from build123d import *

# Parameters (mm, degrees)
SKETCH1_W           = 127
SKETCH1_H           = 101.6
BOSS_EXTRUDE1_DEPTH = 7.62
SKETCH3_W           = 38.1
SKETCH3_H           = 101.6
BOSS_EXTRUDE2_DEPTH = 3.81
SKETCH4_W           = 25.4
SKETCH4_H           = 31.75
CUT_EXTRUDE1_DEPTH  = 7.62
FILLET1_R           = 17.78
BOSS_EXTRUDE3_DEPTH = 10.16
SKETCH6_W           = 1.401774382
SKETCH6_H           = 7.084034581
SKETCH6_W_2         = 1.657965541
SKETCH6_W_3         = 0.723515752
SKETCH6_W_4         = 1.5072414
SKETCH6_W_5         = 1.65796554
SKETCH6_W_6         = 12.660827761
SKETCH6_H_2         = 4.394326049
SKETCH6_W_7         = 12.660827762
BOSS_EXTRUDE4_DEPTH = 5.08
SKETCH7_W           = 0.989162869
SKETCH7_H           = 4.394326049
SKETCH7_W_2         = 1.219468424
CUT_EXTRUDE2_DEPTH  = 5.08
SKETCH8_W           = 20.126718604
SKETCH8_H           = 7.896323228
BOSS_EXTRUDE5_DEPTH = 2.54
SKETCH9_W           = 0.213588314
SKETCH9_H           = 99.880159493
BOSS_EXTRUDE6_DEPTH = 2.54


with BuildPart() as part:
    # Sketch1 → Boss-Extrude1 (new body)
    with BuildSketch(Plane.XY):
        with Locations((63.5, 50.8)):
            Rectangle(SKETCH1_W, SKETCH1_H)
    extrude(amount=BOSS_EXTRUDE1_DEPTH)

    # Sketch3 → Boss-Extrude2 (add)
    with BuildSketch(Plane(origin=(0, 0, 0), x_dir=(-1, 0, 0), z_dir=(0, 0, -1))):
        with Locations((-63.5, 50.8)):
            Rectangle(SKETCH3_W, SKETCH3_H)
    extrude(amount=BOSS_EXTRUDE2_DEPTH)

    # Sketch4 → Cut-Extrude1 (cut)
    with BuildSketch(Plane(origin=(0, 0, 0), x_dir=(-1, 0, 0), z_dir=(0, 0, -1))):
        with Locations((-25.4, 76.835)):
            Rectangle(SKETCH4_W, SKETCH4_H)
        with Locations((-107.95, 76.835)):
            Rectangle(SKETCH4_W, SKETCH4_H)
    extrude(amount=-CUT_EXTRUDE1_DEPTH, mode=Mode.SUBTRACT)

    # Fillet1
    fillet1_edges = [part.edges().sort_by_distance(p)[0] for p in [
        (127, 0, 3.81),
        (0, 0, 3.81),
    ]]
    fillet(fillet1_edges, radius=FILLET1_R)

    # Sketch5 → Boss-Extrude3 (add)
    with BuildSketch(Plane.XZ):
        Polygon((43.18, 7.62), (52.463035847, 23.698689735), (74.536964153, 23.698689735), (83.82, 7.62), align=None)
    extrude(amount=-BOSS_EXTRUDE3_DEPTH)

    # Sketch6 → Boss-Extrude4 (add)
    with BuildSketch(Plane.XZ):
        with Locations((54.433923038, 19.138517409)):
            Rectangle(SKETCH6_W, SKETCH6_H)
        with Locations((58.82755166, 19.138517409)):
            Rectangle(SKETCH6_W_2, SKETCH6_H)
        with Locations((63.515052474, 19.138517409)):
            Rectangle(SKETCH6_W_3, SKETCH6_H)
        with Locations((66.13767245, 19.138517409)):
            Rectangle(SKETCH6_W_4, SKETCH6_H)
        with Locations((69.528965601, 19.138517409)):
            Rectangle(SKETCH6_W_5, SKETCH6_H)
        with Locations((57.99856889, 9.353111302)):
            Rectangle(SKETCH6_W_6, SKETCH6_H_2)
        with Locations((70.659396651, 9.353111302)):
            Rectangle(SKETCH6_W_7, SKETCH6_H_2)
    extrude(amount=BOSS_EXTRUDE4_DEPTH)

    # Sketch7 → Cut-Extrude2 (cut)
    with BuildSketch(Plane.XZ.offset(5.08)):
        with Locations((63.834401336, 9.353111302)):
            Rectangle(SKETCH7_W, SKETCH7_H)
        with Locations((64.938716982, 9.353111302)):
            Rectangle(SKETCH7_W_2, SKETCH7_H)
    extrude(amount=-CUT_EXTRUDE2_DEPTH, mode=Mode.SUBTRACT)

    # Sketch8 → Boss-Extrude5 (add)
    with BuildSketch(Plane.XZ):
        with Locations((62.814636368, 19.241529297)):
            Rectangle(SKETCH8_W, SKETCH8_H)
    extrude(amount=BOSS_EXTRUDE5_DEPTH)

    # Sketch9 → Boss-Extrude6 (add)
    with BuildSketch(Plane.XY.offset(7.62)):
        with Locations((18.943205843, 49.940079747)):
            Rectangle(SKETCH9_W, SKETCH9_H)
    extrude(amount=BOSS_EXTRUDE6_DEPTH)


solid = part.part
Part model, mm, in its own coordinate system. A direction names the side the tool comes from. Coordinates: 2 decimals unless noted, no trailing zeros. Order: outer loops, then holes, each group sorted by start corner. A loop starts at its lowest first (then second) coordinate and runs counter-clockwise, first axis right, second up.
(1) Pull direction X, two halves, no side cores. Call faces 4 (the face through (127, 59, 4)), 5 (the face through (51.668, -3, 9)), 6 (the face through (68.7, -4, 19)): pulls with the +X half, pulls with the -X half, needs draft (parallel to the pull), parting line crosses it, or undercut.
Check sheet entries:
face 4: pulls with the +X half
face 5: pulls with the -X half
face 6: undercut
(2) Slice it at D-D, the plane y = 24. Write the cut outline in (x, z), and give its area (3 significant figures).
Check sheet entries:
outline: (0, 0) - (44.45, 0) - (44.45, -3.81) - (82.55, -3.81) - (82.55, 0) - (127, 0) - (127, 7.62) - (19.05, 7.62) - (19.05, 10.16) - (18.84, 10.16) - (18.84, 7.62) - (0, 7.62) - close
area: 1,110 mm2
(3) Slice it at B-B, the plane x = 23. Write the cut outline in (y, z), and give its area (3 significant figures).
Check sheet entries:
outline: (0, 0) - (60.96, 0) - (60.96, 7.62) - (0, 7.62) - close; (92.71, 0) - (101.6, 0) - (101.6, 7.62) - (92.71, 7.62) - close
area: 532 mm2
(4) Probe L1, parallel to X at y = 74, z = 6.5; L2, parallel to Y at x = 87, z = 4.5; L3, parallel to Y at x = 26.5, z = 1. List the from-to ranges inside material, lowest first.
Check sheet entries:
L1: x = 0 to 12.7, 38.1 to 95.25, 120.65 to 127
L2: y = 0 to 101.6
L3: y = 0 to 60.96, 92.71 to 101.6
(5) Slice it at C-C, the plane z = 5. Write the cut outline in (x, y), and give its area (3 significant figures).
Check sheet entries:
outline: (0, 17.78) arc R17.78 ccw to (17.78, 0) - (109.22, 0) arc R17.78 ccw to (127, 17.78) - (127, 101.6) - (0, 101.6) - close; hole (12.7, 60.96) - (38.1, 60.96) - (38.1, 92.71) - (12.7, 92.71) - close; hole (95.25, 60.96) - (120.65, 60.96) - (120.65, 92.71) - (95.25, 92.71) - close
area: 11,200 mm2
(6) Tool access for faces 1 (the face through (104, 52, 0)), 2 (the face through (59.657, -4, 19)), 3 (the face through (108, 92.71, 4)): list every direction of +Z, -Z, +X, -X, +Y, -Y with a clear straight run to the whole face (end or side of a thin tool).
Check sheet entries:
face 1: -Z, +X, +Y, -Y
face 2: +Z, -Y
face 3: +Z, -Z
(7) Slice it at A-A, the plane y = 87. Write the cut outline in (x, z), and give its area (3 significant figures).
Check sheet entries:
outline: (0, 0) - (12.7, 0) - (12.7, 7.62) - (0, 7.62) - close; (18.84, 7.62) - (19.05, 7.62) - (19.05, 10.16) - (18.84, 10.16) - close; (38.1, 0) - (44.45, 0) - (44.45, -3.81) - (82.55, -3.81) - (82.55, 0) - (95.25, 0) - (95.25, 7.62) - (38.1, 7.62) - close; (120.65, 0) - (127, 0) - (127, 7.62) - (120.65, 7.62) - close
area: 726 mm2
(8) Pin check, flat tips, straight feed: pin 1 Ø12 at (y, z) = (26, 16) entering from -X; pin 2 Ø5.5 at (x, y) = (71, -2.5) entering from +Z; pin 3 Ø2 at (y, z) = (-4, 18) entering from -X; pin 4 Ø12 at (y, z) = (10, 9.5) entering from -X. Stop position of each tip, or through.
Check sheet entries:
pin 1: stops at x = 18.84
pin 2: stops at z = 23.7
pin 3: stops at x = 53.73
pin 4: stops at x = 0.12
